The listing builds one solid part. Answer for the finished solid, in the listing's coordinates (mm). Face numbers are marked on the shaded views. A direction names the side the tool comes from. Coordinates: 2 decimals unless noted, no trailing zeros. Write each loop counter-clockwise with the first axis right and the second up, starting at its lowest first coordinate (ties: lowest second). Pieces come first, ordered by that corner, then holes.
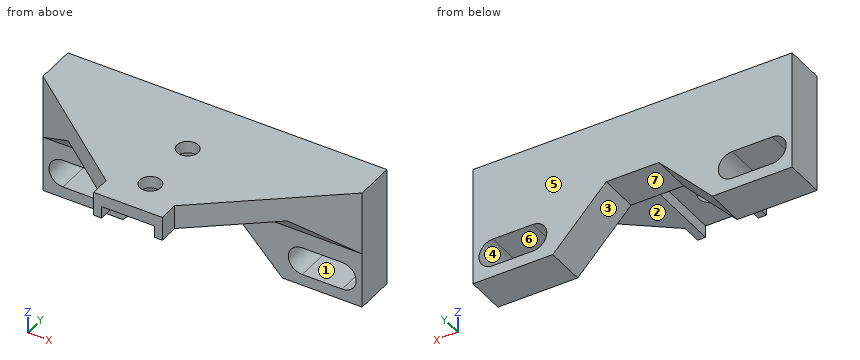
from build123d import *

# Parameters (mm, degrees)
ESQUISSE1_W             = 13.2
ESQUISSE1_H             = 30
ESQUISSE1_W_2           = 2
BOSS_EXTRU_1_DEPTH      = 3
ESQUISSE2_W             = 2
ESQUISSE2_H             = 30
BOSS_EXTRU_2_DEPTH      = 3
BOSS_EXTRU_3_DEPTH      = 10
BOSS_EXTRU_4_DEPTH      = 6
ESQUISSE6_R             = 2.65
ENL_V_MAT_EXTRU_1_DEPTH = 4
ENL_V_MAT_EXTRU_2_DEPTH = 41
CHANFREIN2_SIZE         = 10


with BuildPart() as part:
    # Esquisse1 → Boss.-Extru.1 (new body)
    with BuildSketch(Plane.XY):
        with Locations((-0.437888948, -2.316831683)):
            Rectangle(ESQUISSE1_W, ESQUISSE1_H)
        with Locations((-8.037888948, -2.316831683)):
            Rectangle(ESQUISSE1_W_2, ESQUISSE1_H)
        with Locations((7.162111052, -2.316831683)):
            Rectangle(ESQUISSE1_W_2, ESQUISSE1_H)
    extrude(amount=BOSS_EXTRU_1_DEPTH)

    # Esquisse2 → Boss.-Extru.2 (add)
    with BuildSketch(Plane(origin=(0, 0, 0), x_dir=(-1, 0, 0), z_dir=(0, 0, -1))):
        with Locations((-7.162111052, -2.316831683)):
            Rectangle(ESQUISSE2_W, ESQUISSE2_H)
        with Locations((8.037888948, -2.316831683)):
            Rectangle(ESQUISSE2_W, ESQUISSE2_H)
    extrude(amount=BOSS_EXTRU_2_DEPTH)

    # Esquisse3 → Boss.-Extru.3 (add)
    with BuildSketch(Plane(origin=(0, 12.683168317, 0), x_dir=(1, 0, 0), z_dir=(0, 1, 0))):
        Polygon((19.562111052, 27), (6.162111052, 13), (-7.037888948, 13), (-20.437888948, 27), (-40.437888948, 27), (-40.437888948, -3), (39.562111052, -3), (39.562111052, 27), align=None)
    extrude(amount=BOSS_EXTRU_3_DEPTH)

    # Esquisse5 → Boss.-Extru.4 (add)
    with BuildSketch(Plane.XY.offset(3)):
        Polygon((-9.037888948, 12.683168317), (-40.437888948, 12.683168317), (-9.037888948, -12.316831683), align=None)
        Polygon((8.162111052, -12.316831683), (39.562111052, 12.683168317), (8.162111052, 12.683168317), align=None)
    extrude(amount=-BOSS_EXTRU_4_DEPTH)

    # Esquisse6 → Enlèv. mat.-Extru.1 (cut, through all)
    with BuildSketch(Plane(origin=(0, 0, 0), x_dir=(-1, 0, 0), z_dir=(0, 0, -1))):
        with Locations((0.437888948, 6.683168317)):
            Circle(ESQUISSE6_R)
        with Locations((0.437888948, -8.316831683)):
            Circle(ESQUISSE6_R)
    extrude(amount=-ENL_V_MAT_EXTRU_1_DEPTH, mode=Mode.SUBTRACT)

    # Esquisse7 → Enlèv. mat.-Extru.2 (cut, through all)
    with BuildSketch(Plane(origin=(0, 22.683168317, 0), x_dir=(1, 0, 0), z_dir=(0, 1, 0))):
        with BuildLine():
            Line((-25.437888948, 17.169217815), (-35.437888948, 17.169217815))
            ThreePointArc((-35.437888948, 17.169217815), (-38.937888948, 20.669217815), (-35.437888948, 24.169217815))
            Line((-35.437888948, 24.169217815), (-25.437888948, 24.169217815))
            ThreePointArc((-25.437888948, 24.169217815), (-21.937888948, 20.669217815), (-25.437888948, 17.169217815))
        make_face()
        with BuildLine():
            Line((34.562111052, 17.169217815), (24.562111052, 17.169217815))
            ThreePointArc((24.562111052, 17.169217815), (21.062111052, 20.669217815), (24.562111052, 24.169217815))
            Line((24.562111052, 24.169217815), (34.562111052, 24.169217815))
            ThreePointArc((34.562111052, 24.169217815), (38.062111052, 20.669217815), (34.562111052, 17.169217815))
        make_face()
    extrude(amount=-ENL_V_MAT_EXTRU_2_DEPTH, mode=Mode.SUBTRACT)

    # Chanfrein2
    chanfrein2_edges = [part.edges().sort_by_distance(p)[0] for p in [
        (22.862111052, 12.683168317, -3),
        (-23.737888948, 12.683168317, -3),
    ]]
    chamfer(chanfrein2_edges, length=CHANFREIN2_SIZE)


solid = part.part
Q1. The part is cut by section A-A, the plane y = 20. Write down the section's boundary in (x, z), then the cut area to 3 significant figures.
Answers below:
outline: (-40.44, -27) - (-20.44, -27) - (-7.04, -13) - (6.16, -13) - (19.56, -27) - (39.56, -27) - (39.56, 3) - (-40.44, 3) - close; hole (-35.44, -24.17) - (-25.44, -24.17) arc R3.5 ccw to (-25.44, -17.17) - (-35.44, -17.17) arc R3.5 ccw to start; hole (24.56, -24.17) - (34.56, -24.17) arc R3.5 ccw to (34.56, -17.17) - (24.56, -17.17) arc R3.5 ccw to start
area: 1,810 mm2
Q2. The part is cut by section C-C, the plane x = 23.5. Write down the section's boundary in (y, z), then the cut area to 3 significant figures.
Answers below:
outline: (-0.11, -3) - (2.68, -3) - (12.68, -13) - (12.68, -17.33) - (22.68, -17.33) - (22.68, 3) - (-0.11, 3) - close; (12.68, -27) - (22.68, -27) - (22.68, -24) - (12.68, -24) - close
area: 360 mm2
Q3. The part is cut by section D-D, the plane z = -7.25. Write down the section's boundary in (x, y), then the cut area to 3 significant figures.
Answers below:
outline: (-40.44, 12.68) - (-33.22, 6.93) - (-7.04, 6.93) - (-7.04, 12.68) - (6.16, 12.68) - (6.16, 6.93) - (32.34, 6.93) - (39.56, 12.68) - (39.56, 22.68) - (-40.44, 22.68) - close
area: 1,140 mm2
Q4. Which of the six approach directions +Z, -Z, +X, -X, +Y, -Y give full straight-line access (tool end or side, diameter ignored) to the marked faces 1, 2 and 3?
Answers below:
face 1: +Y, -Y
face 2: -Z, +X, -X, -Y
face 3: -Z, +Y, -Y
Q5. Given pin 1 (6.5 mm diameter, centred on y = 3.5, z = -5.5, fed in from +X); pin 2 (10 mm diameter, centred on x = 5.5, y = -4, fed in from -Z); pin 3 (6.5 mm diameter, centred on x = 2, y = -9.5, fed in from -Z); pin 4 (3 mm diameter, centred on x = -0.44, y = 6.68, fed in from -Z) (3 decimals), each flat-ended and moving along its own axis, determine where each tip first touches the part or whether it passes through.
Answers below:
pin 1: stops at x = 32.11
pin 2: stops at z = -3
pin 3: stops at z = 0
pin 4: passes through
Q6. The part is cut by section B-B, the plane y = -10. Write down the section's boundary in (x, z).
Answers below:
outline: (-11.95, -3) - (-7.04, -3) - (-7.04, 0) - (-2.48, 0) - (-2.48, 3) - (-11.95, 3) - close; (1.61, 0) - (6.16, 0) - (6.16, -3) - (11.07, -3) - (11.07, 3) - (1.61, 3) - close
Q7. Determine the mould class of the marked faces 4, 5, 6 and 7 for opening direction Z: released by +Z, released by -Z, zero draft, split by the parting line, or undercut.
Answers below:
face 4: undercut
face 5: zero draft
face 6: undercut
face 7: released by -Z
Q8. Find the intervals of material crossed by probe 1 along Z at (x, y) = (31, 13); probe 2 along X at (y, z) = (21, -14); probe 3 along Z at (x, y) = (4.5, 14.5), in increasing order.
Answers below:
probe 1: z = -27 to -24.17, -17.17 to 3
probe 2: x = -40.44 to -8, 7.12 to 39.56
probe 3: z = -13 to 3
